Part model, mm, in its own coordinate system. A direction names the side the tool comes from. Round coordinates to 2 decimals unless told otherwise and drop trailing zeros. Write each loop counter-clockwise with the first axis right and the second up, starting at its lowest first coordinate (ties: lowest second). Pieces come first, ordered by that corner, then holes. Notation, with made-up numbers: (39.5, -34.75) -> (90.5, -34.75) arc R32 ccw to (90.5, -3.75) -> close; hole circle Ø7 at (83, 46.25). An arc over 180 degrees is marked (long way). Return JSON: item names as keys, results as strings. Group by question number.
(1) Mould opens along Y. For faces 4 (the flat face through (-15, 0, 6.5)), 5 (the cylindrical face through (2.418, 7.678, -0.035)), 6 (the conical face through (-8.35, -1.85, -3)), 7 (the cylindrical face through (4.95, 15.73, 6.2)) say: +Y half, -Y half, draft (parallel to the pull), parting line (faces both ways), or undercut.
(2) Saw through at A-A (z = -5.5). List the corners of the cut face in (x, y), plus the area to 3 significant figures.
(3) Tool access for faces 1 (the flat face through (21, 2, -9)), 2 (the flat face through (-6, 5, 7)), 3 (the conical face through (-10.527, -2.338, 1.905)): list every direction of +Z, -Z, +X, -X, +Y, -Y with a clear straight run to the whole face (end or side of a thin tool).
(4) Drill centre lines: L1, parallel to X at y = 0, z = 6.1; L2, parallel to Z at x = -21.5, y = -0.5; L3, parallel to X at y = 0, z = 0.6. Where is each one in solid material? Low to high. Write a range as from..to.
(5) Drop flat-ended pins along their axis: pin 1 Ø18.5 at (x, y) = (0, 0) entering from -Z; pin 2 Ø5 at (x, y) = (-15, -8.5) entering from +Z; pin 3 Ø2 at (x, z) = (-5, 3) entering from -Y. Give the stop position or say it passes through.
from build123d import *

# Parameters (mm, degrees)
FILLET1_R = 1


with BuildPart() as part:
    # Sketch1 → Revolve1 (revolve)
    with BuildSketch(Plane(origin=(0, 0, 0), x_dir=(0, 0, -1), z_dir=(1, 0, 0))):
        with BuildLine():
            Line((-2.5, 8.05), (2.5, 8.05))
            Line((2.5, 8.05), (10.5, 16.05))
            Line((10.5, 16.05), (10.5, 26.916438469))
            Line((10.5, 26.916438469), (9, 26.916438469))
            Line((9, 26.916438469), (9, 20.916438469))
            Line((9, 20.916438469), (1.638304089, 10.402847127))
            ThreePointArc((1.638304089, 10.402847127), (0, 9.55), (-1.638304089, 10.402847127))
            Line((-1.638304089, 10.402847127), (-5.9, 16.489179649))
            Line((-5.9, 16.489179649), (-6.5, 16.489179649))
            Line((-6.5, 16.489179649), (-6.5, 14.489179649))
            ThreePointArc((-6.5, 14.489179649), (-6.625190798, 11.284822592), (-7, 8.1))
            Line((-7, 8.1), (-7, 7.5))
            Line((-7, 7.5), (-3.05, 7.5))
            Line((-3.05, 7.5), (-2.5, 8.05))
        make_face()
    revolve(axis=Axis((0, 0, 162.721569491), (0, 0, -1)))

    # Fillet1
    fillet1_edges = [part.edges().sort_by_distance(p)[0] for p in [
        (0, -26.916438469, -9),
    ]]
    fillet(fillet1_edges, radius=FILLET1_R)


solid = part.part
Computed values:
{
 "1": {"face 4": "draft", "face 5": "undercut", "face 6": "undercut", "face 7": "parting line"},
 "2": {"outline": "circle Ø31.84 at (0, 0); hole circle Ø22.1 at (0, 0)", "area": "412 mm2"},
 "3": {"face 1": "+Z", "face 2": "+Z, +X, -X, +Y, -Y", "face 3": "none"},
 "4": {"L1": "-16.49..-7.5, 7.5..16.49", "L2": "-10.5..-9", "L3": "-9.64..-8.05, 8.05..9.64"},
 "5": {"pin 1": "z = -3.7", "pin 2": "z = 6.5", "pin 3": "y = -12.88"}
}
